Read the model definition and answer for the solid it produces. Units are mm, in the model's axes. A direction names the side the tool comes from. Coordinates: 2 decimals unless noted, no trailing zeros. Loops run counter-clockwise (first coordinate to the right, second up) from the corner with the lowest first, then second, coordinate; pieces in that order, holes last. Notation, with made-up numbers: (-13, 48.5) - (24, 48.5) arc R25 cw to (24, 84.5) - close; hole circle Ø6 at (63, 19). An arc over 180 degrees is marked (long way). One line per item, written item: value. Start each with the question number.
from build123d import *

# Parameters (mm, degrees)
SKETCH_1_W      = 20
SKETCH_1_H      = 60
SKETCH_1_R      = 1.5
SKETCH_1_W_2    = 10
SKETCH_1_H_2    = 35
EXTRUDE_1_DEPTH = 3
CHAMFER_1_SIZE  = 3
FILLET_1_R      = 3


with BuildPart() as part:
    # 草图1 → 凸台-拉伸1 (new body)
    with BuildSketch(Plane(origin=(0, 0, 0), x_dir=(1, 0, 0), z_dir=(0, 1, 0))):
        Rectangle(SKETCH_1_W, SKETCH_1_H)
        with Locations(Location((-4, 26, 0), (0, 0, 270))):
            Circle(SKETCH_1_R, mode=Mode.SUBTRACT)
        with Locations(Location((4, 26, 0), (0, 0, 90))):
            Circle(SKETCH_1_R, mode=Mode.SUBTRACT)
        with Locations(Location((4, -26, 0), (0, 0, 270))):
            Circle(SKETCH_1_R, mode=Mode.SUBTRACT)
        with Locations(Location((-4, -26, 0), (0, 0, 90))):
            Circle(SKETCH_1_R, mode=Mode.SUBTRACT)
        Rectangle(SKETCH_1_W_2, SKETCH_1_H_2, mode=Mode.SUBTRACT)
    extrude(amount=EXTRUDE_1_DEPTH)

    # 倒角1
    chamfer_1_edges = [part.edges().sort_by_distance(p)[0] for p in [
        (5, 1.5, 17.5),
        (5, 1.5, -17.5),
        (-5, 1.5, -17.5),
        (-5, 1.5, 17.5),
    ]]
    chamfer(chamfer_1_edges, length=CHAMFER_1_SIZE)

    # 圆角1
    fillet_1_edges = [part.edges().sort_by_distance(p)[0] for p in [
        (10, 1.5, 30),
        (-10, 1.5, 30),
        (-10, 1.5, -30),
        (10, 1.5, -30),
    ]]
    fillet(fillet_1_edges, radius=FILLET_1_R)


solid = part.part
1) For faces 1 (the flat face through (5, 1, 0)), 2 (the cylindrical face through (-9.14, 1.52, 29.1)), determine the directions among +Z, -Z, +X, -X, +Y, -Y from which every point of the face is accessible in a straight line to the end or side of a thin tool.
2) Section A-A, the plane z = 26 is taken. Determine the outline of the cut face in (x, y), and give its area (3 significant figures).
3) Section C-C, the plane z = -7 is taken. Determine the outline of the cut face in (x, y), and give its area (3 significant figures).
4) Determine the mould class of faces 3 (the flat face through (-10, 1, 0)), 4 (the flat face through (0, 1, 30)), 5 (the cylindrical face through (-4.07, 1.48, 27.5)) for opening direction X: released by +X, released by -X, zero draft, split by the parting line, or undercut.
5) Section B-B, the plane x = -4 is taken. Determine the outline of the cut face in (y, z), and give its area (3 significant figures).
6) Section D-D, the plane y = 1.35 is taken. Determine the outline of the cut face in (x, z).
7) Straight lines are drawn through the part: L1, parallel to X at y = 1.4, z = -26; L2, parallel to X at y = 1.6, z = 12.5; L3, parallel to Z at x = -2, y = 1.55. For each, find the intervals that lie inside material, in ascending order.
Answer below:
1. face 1: +Y, -Y
1. face 2: +Z, -X, +Y, -Y
2. outline: (-10, 0) - (-5.5, 0) - (-5.5, 3) - (-10, 3) - close; (-2.5, 0) - (2.5, 0) - (2.5, 3) - (-2.5, 3) - close; (5.5, 0) - (10, 0) - (10, 3) - (5.5, 3) - close
2. area: 42.0 mm2
3. outline: (-10, 0) - (-5, 0) - (-5, 3) - (-10, 3) - close; (5, 0) - (10, 0) - (10, 3) - (5, 3) - close
3. area: 30.0 mm2
4. face 3: released by -X
4. face 4: zero draft
4. face 5: undercut
5. outline: (0, -30) - (3, -30) - (3, -27.5) - (0, -27.5) - close; (0, -24.5) - (3, -24.5) - (3, -15.5) - (0, -15.5) - close; (0, 15.5) - (3, 15.5) - (3, 24.5) - (0, 24.5) - close; (0, 27.5) - (3, 27.5) - (3, 30) - (0, 30) - close
5. area: 69.0 mm2
6. outline: (-10, -27) arc R3 ccw to (-7, -30) - (7, -30) arc R3 ccw to (10, -27) - (10, 27) arc R3 ccw to (7, 30) - (-7, 30) arc R3 ccw to (-10, 27) - close; hole circle Ø3 at (-4, -26); hole circle Ø3 at (-4, 26); hole (-5, -14.5) - (-2, -17.5) - (2, -17.5) - (5, -14.5) - (5, 14.5) - (2, 17.5) - (-2, 17.5) - (-5, 14.5) - close; hole circle Ø3 at (4, -26); hole circle Ø3 at (4, 26)
7. L1: -10 to -5.5, -2.5 to 2.5, 5.5 to 10
7. L2: -10 to -5, 5 to 10
7. L3: -30 to -17.5, 17.5 to 30
